```python
from build123d import *

# Parameters (mm, degrees)
BOSS_EXTRUDE1_DEPTH = 20
BOSS_EXTRUDE2_START = -20
SKETCH4_R           = 10
BOSS_EXTRUDE2_DEPTH = 23


with BuildPart() as part:
    # Sketch1 → Boss-Extrude1 (new body)
    with BuildSketch(Plane.XY):
        Polygon((0, 0), (0, -27.999047944), (-3, -27.999047944), (-3, -2.999047944), (-31.907622925, -2.999047944), (-31.907622925, 37.000952056), (-28.907622925, 37.000952056), (-28.907622925, 0), align=None)
    extrude(amount=BOSS_EXTRUDE1_DEPTH)

    # Sketch4 → Boss-Extrude2 (add)
    with BuildSketch(Plane(origin=(0, 0, 0), x_dir=(-1, 0, 0), z_dir=(0, 0, -1)).offset(BOSS_EXTRUDE2_START)):
        with Locations((1.5, -24.299047944)):
            Circle(SKETCH4_R)
    extrude(amount=BOSS_EXTRUDE2_DEPTH)


solid = part.part
```
The listing builds one solid part. Answer for the finished solid, in the listing's coordinates (mm). A direction names the side the tool comes from. Give positions to 0.01 mm unless a question says otherwise; leave off trailing zeros. Write each loop counter-clockwise with the first axis right and the second up, starting at its lowest first coordinate (ties: lowest second). Pieces come first, ordered by that corner, then holes. Notation, with made-up numbers: M -25.5,58.25 L 32.5,58.25 A21 ccw 32.5,86.25 Z; hole C 31,81 d1. An arc over 180 degrees is marked long. Write each question's results on one line, items separated by ' | '.
Q1. A tool of negligible diameter and unlimited length cuts with its end or side. For faces 4 (the flat face through (-3, -9, 10)), 5 (the flat face through (-1, -24, -3)), 6 (the flat face through (-28.908, 19, 10)), from which of +Z, -Z, +X, -X, +Y, -Y can it reach the whole face along a straight path? Write none if from no direction.
Output values:
face 4: +Z, -Z, -X | face 5: -Z, +X, -X, +Y, -Y | face 6: +Z, -Z, +X, +Y
Q2. Section C-C, the plane x = -1.5 is taken. Write down the section's boundary in (y, z).
Output values:
outline: M -34.3,-3 L -14.3,-3 L -14.3,0 L 0,0 L 0,20 L -34.3,20 Z
Q3. Flat-ended cylindrical pins translate along their axes: P1, Ø11.5, axis at y = -7.5, z = 13, coming from the +X side; P2, Ø5, axis at y = -13.5, z = 17.5, coming from the +X side; P3, Ø12, axis at x = 3, z = 12.5, coming from the +Y side; P4, Ø16, axis at x = -14, y = 19, coming from the -Z side. Find the tip coordinate at first contact, or state that the pin passes through.
Output values:
P1: x = 0 | P2: x = 4.08 | P3: y = 0 | P4: through
Q4. Consider L1, parallel to Y at x = -24, z = 11.5; L2, parallel to Z at x = -30, y = 1; L3, parallel to X at y = 15.5, z = 9.5. Determine where each line is inside the solid, lowest interval first. Write a range as from..to.
Output values:
L1: -3..0 | L2: 0..20 | L3: -31.91..-28.91
Q5. For a pull along Y with two mould halves and no side action, classify faces 1 (the flat face through (-17, -2.999, 10)), 2 (the flat face through (-30, 37.001, 10)), 3 (the flat face through (0, -7, 10)) as released by +Y, released by -Y, zero draft, split by the parting line, or undercut.
Output values:
face 1: undercut | face 2: released by +Y | face 3: zero draft
Q6. Section B-B, the plane z = 8 is taken. Write down the section's boundary in (x, y), then the cut area to 3 significant figures.
Output values:
outline: M -31.91,-3 L -3,-3 L -3,-14.41 A10 ccw long 0,-14.41 L 0,0 L -28.91,0 L -28.91,37 L -31.91,37 Z | area: 555 mm2
Q7. Section D-D, the plane y = 1.5 is taken. Write down the section's boundary in (x, z), then the cut area to 3 significant figures.
Output values:
outline: M -31.91,0 L -28.91,0 L -28.91,20 L -31.91,20 Z | area: 60.0 mm2
Q8. Section A-A, the plane x = -6 is taken. Write down the section's boundary in (y, z).
Output values:
outline: M -33.23,-3 L -15.37,-3 L -15.37,20 L -33.23,20 Z; M -3,0 L 0,0 L 0,20 L -3,20 Z
